Check sheet for the modelled part. Datum: model origin and axes. Units: mm. Face numbers are marked on the shaded views. A direction names the side the tool comes from. Coordinates: 2 decimals unless noted, no trailing zeros. Order: outer loops, then holes, each group sorted by start corner. A loop starts at its lowest first (then second) coordinate and runs counter-clockwise, first axis right, second up.
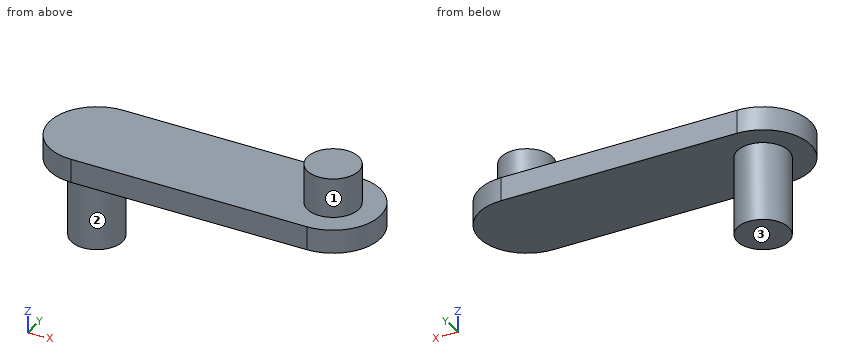
from build123d import *

# Parameters (mm, degrees)
Y_KSEKLIK_EKSTR_ZYON1_DEPTH = 3
IZIM2_R                     = 3.25
Y_KSEKLIK_EKSTR_ZYON2_DEPTH = 5
IZIM3_R                     = 3.25
Y_KSEKLIK_EKSTR_ZYON3_DEPTH = 10


with BuildPart() as part:
    # Çizim1 → Yükseklik-Ekstrüzyon1 (new body)
    with BuildSketch(Plane.XY):
        with BuildLine():
            Line((-15, 6), (15, 6))
            ThreePointArc((15, 6), (21, 0), (15, -6))
            Line((15, -6), (-15, -6))
            ThreePointArc((-15, -6), (-21, 0), (-15, 6))
        make_face()
    extrude(amount=Y_KSEKLIK_EKSTR_ZYON1_DEPTH)

    # Çizim2 → Yükseklik-Ekstrüzyon2 (add)
    with BuildSketch(Plane.XY.offset(3)):
        with Locations((15, 0)):
            Circle(IZIM2_R)
    extrude(amount=Y_KSEKLIK_EKSTR_ZYON2_DEPTH)

    # Çizim3 → Yükseklik-Ekstrüzyon3 (add)
    with BuildSketch(Plane(origin=(0, 0, 0), x_dir=(-1, 0, 0), z_dir=(0, 0, -1))):
        with Locations(Location((15, 0, 0), (0, 0, 180))):
            Circle(IZIM3_R)
    extrude(amount=Y_KSEKLIK_EKSTR_ZYON3_DEPTH)


solid = part.part
(1) Cross-section at B-B (z = 6.5). Enter the section's corners in (x, y), and give its area (3 significant figures).
Filled in:
outline: circle Ø6.5 at (15, 0)
area: 33.2 mm2
(2) Tool access check on the marked faces 1, 2 and 3. Record the directions out of +Z, -Z, +X, -X, +Y, -Y that give a thin tool (end or side, any length) a straight path to the whole face; none if there is none.
Filled in:
face 1: +Z
face 2: -Z
face 3: -Z, +X, -X, +Y, -Y
(3) Cross-section at C-C (x = 11). Enter the section's corners in (y, z).
Filled in:
outline: (-6, 0) - (6, 0) - (6, 3) - (-6, 3) - close
(4) Thickness scan on probe 1 along Z at (x, y) = (-2, -4); probe 2 along X at (y, z) = (-0.25, -7); probe 3 along X at (y, z) = (-1, 5.25). Record the ranges inside material, lowest first.
Filled in:
probe 1: z = 0 to 3
probe 2: x = -18.24 to -11.76
probe 3: x = 11.91 to 18.09
(5) Go/stop test with flat-tipped pins: P1, Ø6, axis at x = -0.5, y = -3, coming from the -Z side; P2, Ø3, axis at x = -11, z = -6.5, coming from the -Y side; P3, Ø1, axis at y = 0, z = -5, coming from the +X side. Record where each tip stops, or that it passes through.
Filled in:
P1: stops at z = 0
P2: stops at y = -2.08
P3: stops at x = -11.75
(6) Cross-section at A-A (y = 0). Enter the section's corners in (x, z).
Filled in:
outline: (-21, 0) - (-18.25, 0) - (-18.25, -10) - (-11.75, -10) - (-11.75, 0) - (21, 0) - (21, 3) - (18.25, 3) - (18.25, 8) - (11.75, 8) - (11.75, 3) - (-21, 3) - close
(7) Cross-section at D-D (y = -2.25). Enter the section's corners in (x, z).
Filled in:
outline: (-20.56, 0) - (-17.35, 0) - (-17.35, -10) - (-12.65, -10) - (-12.65, 0) - (20.56, 0) - (20.56, 3) - (17.35, 3) - (17.35, 8) - (12.65, 8) - (12.65, 3) - (-20.56, 3) - close
